Geometry check sheet. Reference: the model listing, model coordinates, mm. Give positions to 0.01 mm unless a question says otherwise; leave off trailing zeros. Write each loop counter-clockwise with the first axis right and the second up, starting at its lowest first coordinate (ties: lowest second). Pieces come first, ordered by that corner, then holes. Notation, with made-up numbers: M 22,46 L 29,46 A28 ccw 29,84 Z; hole C -29,-37 d3. An arc over 180 degrees is marked long. One line per item, written item: value. Start each with the question number.
1. Cross-section at A-A on x = -42.5. Record the cut outline in (y, z).
2. Release check for a two-part mould opening along X. For faces 1 (the face through (-129.24, 42.14, 1.48)), 2 (the face through (-31, -7, 3)), 3 (the face through (-119.762, 22.176, 1.479)) record: pulls with the +X half, pulls with the -X half, needs draft (parallel to the pull), parting line crosses it, or undercut.
3. Gauge pin test, flat end, axial feed: pin 1 (2.5 mm diameter, centred on x = 68.39, y = -47.84, fed in from -Z). Record the tip position at first contact, or that the pin passes through.
4. Scan lines: line 1 (Y direction, x = -93, z = 2.65); line 2 (Y direction, x = -97, z = 2.05); line 3 (Y direction, x = -138.3, z = 1.3). Record each from-to range of solid material in increasing order.
5. Cross-section at B-B on z = 1.35. Count the separate pieces of the cut face and the enclosed holes in it, then the cut area to 3 significant figures.
from build123d import *

# Parameters (mm, degrees)
SKETCH1_R           = 2
SKETCH1_R_2         = 16
SKETCH1_R_3         = 2.25
SKETCH1_R_4         = 5.5
SKETCH1_R_5         = 1.75
SKETCH1_R_6         = 8.75
BOSS_EXTRUDE1_DEPTH = 3
SKETCH2_R           = 1.5
CUT_EXTRUDE1_DEPTH  = 190.515777006


with BuildPart() as part:
    # Sketch1 → Boss-Extrude1 (new body)
    with BuildSketch(Plane.XY):
        with BuildLine():
            ThreePointArc((-137.970351553, -33.480224156), (-126.431132561, -39.888203569), (-124.422839539, -52.93360637))
            ThreePointArc((-124.422839539, -52.93360637), (-124.888175134, -64.31939994), (-119.594822483, -74.410646153))
            Line((-119.594822483, -74.410646153), (-92.540517723, -103.740413224))
            ThreePointArc((-92.540517723, -103.740413224), (-82.119700521, -108.557935129), (-71.344567605, -104.595807028))
            Line((-71.344567605, -104.595807028), (-37.221129556, -73.119733925))
            ThreePointArc((-37.221129556, -73.119733925), (-32.538343047, -69.892896145), (-27.140055215, -68.104192696))
            Line((-27.140055215, -68.104192696), (68.925058584, -50.795851294))
            ThreePointArc((68.925058584, -50.795851294), (82.107908339, -44.886103489), (91, -33.5))
            ThreePointArc((91, -33.5), (96.805715124, 7.17766304), (80.26119478, 44.789595257))
            ThreePointArc((80.26119478, 44.789595257), (69.434281248, 53.01522195), (56.08825014, 55.616461034))
            Line((56.08825014, 55.616461034), (-113.612396892, 49.485657177))
            ThreePointArc((-113.612396892, 49.485657177), (-129.404309407, 41.953313258), (-134.705774542, 25.279526249))
            ThreePointArc((-134.705774542, 25.279526249), (-136.343375771, 16.802270376), (-142.382746132, 10.632050724))
            ThreePointArc((-142.382746132, 10.632050724), (-155.099864059, -8.058287742), (-147.542861296, -29.364285714))
            ThreePointArc((-147.542861296, -29.364285714), (-143.125485566, -32.280163581), (-137.970351553, -33.480224156))
        make_face()
        with Locations((-81.514845762, -93.570135067)):
            Circle(SKETCH1_R, mode=Mode.SUBTRACT)
        with Locations((-103.42383694, -59.494238188)):
            Circle(SKETCH1_R_2, mode=Mode.SUBTRACT)
        with Locations((-138.3, -22.75)):
            Circle(SKETCH1_R, mode=Mode.SUBTRACT)
        with Locations((-138.3, -5.25)):
            Circle(SKETCH1_R, mode=Mode.SUBTRACT)
        with Locations((-68.3, -21.5)):
            Circle(SKETCH1_R_3, mode=Mode.SUBTRACT)
        with Locations((-74.1, 1.7)):
            Circle(SKETCH1_R_3, mode=Mode.SUBTRACT)
        with Locations((-65.4, 20.2)):
            Circle(SKETCH1_R_3, mode=Mode.SUBTRACT)
        with Locations((18.5, -8.7)):
            Circle(SKETCH1_R_3, mode=Mode.SUBTRACT)
        with Locations((8.1, 8.2)):
            Circle(SKETCH1_R_3, mode=Mode.SUBTRACT)
        with Locations((75.9, -21.8)):
            Circle(SKETCH1_R_3, mode=Mode.SUBTRACT)
        with Locations((40.017782272, 0)):
            Circle(SKETCH1_R_4, mode=Mode.SUBTRACT)
        with Locations((78, -0.1)):
            Circle(SKETCH1_R_3, mode=Mode.SUBTRACT)
        with Locations((73, 22.4)):
            Circle(SKETCH1_R_3, mode=Mode.SUBTRACT)
        with Locations((-114.213840088, 40.424858245)):
            Circle(SKETCH1_R_5, mode=Mode.SUBTRACT)
        with Locations((-111.422396488, 14.575141755)):
            Circle(SKETCH1_R_5, mode=Mode.SUBTRACT)
        with Locations((-125.742976533, 26.1042782)):
            Circle(SKETCH1_R_5, mode=Mode.SUBTRACT)
        with Locations((-112.818118288, 27.5)):
            Circle(SKETCH1_R_6, mode=Mode.SUBTRACT)
        with Locations((-99.893260043, 28.8957218)):
            Circle(SKETCH1_R_5, mode=Mode.SUBTRACT)
    extrude(amount=BOSS_EXTRUDE1_DEPTH)

    # Sketch2 → Cut-Extrude1 (cut, through all)
    with BuildSketch(Plane.XY.offset(3)):
        with Locations((56.196560986, 52.618416878)):
            Circle(SKETCH2_R)
        with Locations((-23.803439014, 49.728243404)):
            Circle(SKETCH2_R)
        with Locations((-103.803439014, 46.83806993)):
            Circle(SKETCH2_R)
        with Locations((68.393104802, -47.843390427)):
            Circle(SKETCH2_R)
        with Locations((-10.390547842, -62.038078831)):
            Circle(SKETCH2_R)
        with Locations((-152.133709173, -14)):
            Circle(SKETCH2_R)
        with Locations((-89.174200485, -76.232767235)):
            Circle(SKETCH2_R)
    extrude(amount=-CUT_EXTRUDE1_DEPTH, mode=Mode.SUBTRACT)


solid = part.part
Report:
1. outline: M -77.99,0 L 52.05,0 L 52.05,3 L -77.99,3 Z
2. face 1: pulls with the -X half
2. face 2: needs draft
2. face 3: undercut
3. pin 1: passes through
4. line 1: y = -103.24 to -71.63, -47.36 to 50.23
4. line 2: y = -98.91 to -74.15, -44.84 to 50.09
4. line 3: y = -33.46 to -24.75, -20.75 to -7.25, -3.25 to 13.93
5. separate pieces: 1
5. enclosed holes: 25
5. area: 27,000 mm^2
